```python
from build123d import *

# Parameters (mm, degrees)
F0_W     = 105.3343974054
F0_H     = 65.4578059912
F1_DEPTH = 25
F3_D     = 8.5
F4_T     = -2.5


with BuildPart() as f1:
    # F0 (on Front) → F1 (new body)
    with BuildSketch(Plane.XZ):
        with Locations((3.6365445703, 2.0063705742)):
            Rectangle(F0_W, F0_H)
    extrude(amount=F1_DEPTH)

    # F3 (through all)
    with Locations(Plane.XZ.offset(25)):
        with Locations((-22.0700632781, 16.4271499962), (0, 22.4462598562), (18.8097134233, 27.7129784226), (43.8893288374, 16.4271499962), (-28.8415607065, -12.6652074978), (0, 0), (27.838377282, -16.6779458523)):
            Hole(F3_D / 2)

    # F4
    f4_openings = [f1.faces().sort_by_distance(p)[0] for p in [
        (-47.79049, -25, 2.006371),
    ]]
    offset(amount=F4_T, openings=f4_openings)


solid = f1.part
```
Can you work these out from the model? Positions are in its coordinate system, mm. A direction names the side the tool comes from. Round coordinates to 2 decimals unless told otherwise and drop trailing zeros. Loops run counter-clockwise (first coordinate to the right, second up) from the corner with the lowest first, then second, coordinate; pieces in that order, holes last. Notation, with made-up numbers: (57, 10) -> (93, 10) arc R17 cw to (93, 15) -> close; hole circle Ø3 at (25.5, -21). An arc over 180 degrees is marked (long way). One line per item, written item: value. Start each with the question number.
1. If we section it at B-B, the plane z = 0: Write out the boundary of the cut face in (x, y).
2. For pin 1 (12 mm diameter, centred on x = -20, z = -11, fed in from -Y); pin 2 (1 mm diameter, centred on x = 19.5, z = -2.5, fed in from -Y), each with a flat end and sliding along its axis, tell me the tip position at first contact or that it passes through.
3. If we section it at A-A, the plane x = 0: Write out the boundary of the cut face in (y, z), then the cut area to 3 significant figures.
4. For faces 4 (the cylindrical face through (-25.185, -13.592, 10.439)), 5 (the cylindrical face through (-2.285, -12.325, 3.584)), which set-ups out of +Z, -Z, +X, -X, +Y, -Y let a thin tool reach every point of the face, with its end or its side?
5. If we section it at C-C, the plane y = -5.5: Give the number of separate pieces and of enclosed holes in the cut face, then the cut area to 3 significant figures.
6. If I drill on probe 1 along X at (y, z) = (-17.5, -12); probe 2 along Z at (x, y) = (-1, -21.25); probe 3 along Z at (x, y) = (-12.5, -16.75), over which ranges is the centre line in solid material (lowest first)?
7. If we mould it in two halves opening along X, with no side actions, what happens to faces 1 (the cylindrical face through (19.027, -13.593, 20.966)), 2 (the flat face through (32.24, -25, -16.58)), 3 (the flat face through (-49.031, -12, 2))? For each: pulls with the +X half, pulls with the -X half, needs draft (parallel to the pull), parting line crosses it, or undercut.
Calculated:
1. outline: (-49.03, -25) -> (-46.53, -25) -> (-46.53, -2.5) -> (-6.75, -2.5) -> (-6.75, -25) -> (-4.25, -25) -> (-4.25, 0) -> (-49.03, 0) -> close; (4.25, -25) -> (6.75, -25) -> (6.75, -2.5) -> (53.8, -2.5) -> (53.8, -25) -> (56.3, -25) -> (56.3, 0) -> (4.25, 0) -> close
2. pin 1: stops at y = -25
2. pin 2: stops at y = -2.5
3. outline: (-25, -30.72) -> (0, -30.72) -> (0, -4.25) -> (-25, -4.25) -> (-25, -6.75) -> (-2.5, -6.75) -> (-2.5, -28.22) -> (-25, -28.22) -> close; (-25, 4.25) -> (0, 4.25) -> (0, 18.2) -> (-25, 18.2) -> (-25, 15.7) -> (-2.5, 15.7) -> (-2.5, 6.75) -> (-25, 6.75) -> close; (-25, 26.7) -> (0, 26.7) -> (0, 34.74) -> (-25, 34.74) -> (-25, 32.24) -> (-2.5, 32.24) -> (-2.5, 29.2) -> (-25, 29.2) -> close
3. area: 459 mm²
4. face 4: -Y
4. face 5: +Y, -Y
5. separate pieces: 7
5. enclosed holes: 8
5. area: 1,420 mm²
6. probe 1: x = -49.03 to -46.53, -35.56 to -33.04, -24.64 to -22.12, 22.97 to 32.7, 53.8 to 56.3
6. probe 2: z = -30.72 to -28.22, -6.68 to -4.13, 4.13 to 6.68, 15.77 to 18.32, 26.58 to 29.12, 32.24 to 34.74
6. probe 3: z = -30.72 to -28.22, 32.24 to 34.74
7. face 1: undercut
7. face 2: needs draft
7. face 3: pulls with the -X half
